Autodesk Inventor part; units mm, degrees
ref_plane "YZ Plane" through (0, 0, 0) normal (1, 0, 0) x (0, 1, 0)
ref_plane "XZ Plane" through (0, 0, 0) normal (0, 1, 0) x (-1, 0, 0)
ref_plane "XY Plane" through (0, 0, 0) normal (0, 0, 1) x (1, 0, 0)
sketch "Sketch1" plane through (0, 0, 0) normal (1, 0, 0) x (0, 1, 0)
  line L0 (0, 12.7) -> (0, -12.7)
  line L1 (0, 12.7) -> (25.4, 12.7)
  line L2 (0, -12.7) -> (25.4, -12.7)
  line L3 (25.4, 9.525) -> (3.175, 9.525)
  line L4 (3.175, 9.525) -> (3.175, -9.525)
  line L5 (3.175, -9.525) -> (25.4, -9.525)
  line L6 (25.4, 12.7) -> (25.4, 9.525)
  line L7 (25.4, -9.525) -> (25.4, -12.7)
  point P0 (0, 0)
  point P1 (0, 0)
  dimension "d0" = 25.4
  dimension "d1" = 25.4
  dimension "d2" = 25.4
  dimension "d3" = 3.175
extrude "Extrusion1" add sketch "Sketch1" along normal mid plane 64
sketch "Sketch2" plane through (-32, 3.175, 9.525) normal (0, 1, 0) x (1, 0, 0)
  circle A0 centre (4.5, 9.525) radius 3
  line L0 (0, 0) -> (0, 19.05) construction
  line L1 (0, 19.05) -> (64, 19.05) construction
  circle A1 centre (15.5, 9.525) radius 3
  circle A2 centre (26.5, 9.525) radius 3
  circle A3 centre (37.5, 9.525) radius 3
  circle A4 centre (48.5, 9.525) radius 3
  circle A5 centre (59.5, 9.525) radius 3
  point P0 (32, 9.525)
  point P1 (0, 9.525)
  point P2 (0, 9.525)
  dimension "d6" = 6
  dimension "d7" = 4.5
  dimension "d10" = 11
extrude "Extrusion2" cut sketch "Sketch2" against normal through all
sketch "Sketch3" plane through (-32, 0, 12.7) normal (0, 0, 1) x (1, 0, 0)
  line L0 (0, 3.175) -> (64, 3.175) construction
  line L1 (64, 25.4) -> (64, 3.175) construction
  line L2 (0, 25.4) -> (64, 25.4) construction
  line L3 (0, 3.175) -> (0, 25.4) construction
  circle A0 centre (4.5, 15.625) radius 3
  circle A1 centre (15.5, 15.625) radius 3
  circle A2 centre (26.5, 15.625) radius 3
  circle A3 centre (37.5, 15.625) radius 3
  circle A4 centre (48.5, 15.625) radius 3
  circle A5 centre (59.5, 15.625) radius 3
  point P0 (32, 0)
  dimension "d17" = 6
  dimension "d18" = 12.45
  dimension "d19" = 4.5
  dimension "d22" = 11
extrude "Extrusion3" cut sketch "Sketch3" against normal through all
properties part number "ArmSupport_C-Channel"
CAD build for the part. Positions are in the model's coordinates, mm. A direction names the side the tool comes from. Round coordinates to 2 decimals unless told otherwise and drop trailing zeros. Order: outer loops, then holes, each group sorted by start corner. A loop starts at its lowest first (then second) coordinate and runs counter-clockwise, first axis right, second up. Notation, with made-up numbers: (80, 14) -> (120, 14) arc R8 ccw to (120, 28) -> close; hole circle Ø9 at (87.25, 62.5). An arc over 180 degrees is marked (long way). Write item = value, one per line.
(1) Cut at A-A (z = 0). Write the cut outline in (x, y) (3 decimals).
Answers follow:
outline = (-32, 0) -> (-30.5, 0) -> (-30.5, 3.175) -> (-32, 3.175) -> close; (-24.5, 0) -> (-19.5, 0) -> (-19.5, 3.175) -> (-24.5, 3.175) -> close; (-13.5, 0) -> (-8.5, 0) -> (-8.5, 3.175) -> (-13.5, 3.175) -> close; (-2.5, 0) -> (2.5, 0) -> (2.5, 3.175) -> (-2.5, 3.175) -> close; (8.5, 0) -> (13.5, 0) -> (13.5, 3.175) -> (8.5, 3.175) -> close; (19.5, 0) -> (24.5, 0) -> (24.5, 3.175) -> (19.5, 3.175) -> close; (30.5, 0) -> (32, 0) -> (32, 3.175) -> (30.5, 3.175) -> close
(2) Drill centre lines: L1, parallel to Z at x = -25, y = 12.5 (3 decimals); L2, parallel to Y at x = -27.5, z = -12 (3 decimals); L3, parallel to Y at x = -26, z = -3.5 (3 decimals). Where is each one in solid material? Low to high.
Answers follow:
L1 = -12.7 to -9.525, 9.525 to 12.7
L2 = 0 to 12.625, 18.625 to 25.4
L3 = 0 to 3.175
(3) Cut at D-D (x = 21.5). Write the cut outline in (y, z) (3 decimals).
Answers follow:
outline = (0, -12.7) -> (25.4, -12.7) -> (25.4, -9.525) -> (3.175, -9.525) -> (3.175, 9.525) -> (25.4, 9.525) -> (25.4, 12.7) -> (0, 12.7) -> close
(4) Pull direction X, two halves, no side cores. Call faces 1 (the flat face through (0, 13, -12.7)), 2 (the flat face through (-32, 2, 0)), 3 (the flat face through (32, 2, 0)), 4 (the cylindrical face through (-19.5, 1.6, -0.1)): +X half, -X half, draft (parallel to the pull), parting line (faces both ways), or undercut.
Answers follow:
face_1 = draft
face_2 = -X half
face_3 = +X half
face_4 = undercut
(5) Cut at B-B (x = -5.5). Write the cut outline in (y, z) (3 decimals), plus the area to 3 significant figures.
Answers follow:
outline = (0, -12.7) -> (12.625, -12.7) -> (12.625, -9.525) -> (3.175, -9.525) -> (3.175, -3) -> (0, -3) -> close; (0, 3) -> (3.175, 3) -> (3.175, 9.525) -> (12.625, 9.525) -> (12.625, 12.7) -> (0, 12.7) -> close; (18.625, -12.7) -> (25.4, -12.7) -> (25.4, -9.525) -> (18.625, -9.525) -> close; (18.625, 9.525) -> (25.4, 9.525) -> (25.4, 12.7) -> (18.625, 12.7) -> close
area = 165 mm²
(6) Flat gauge pins, fed straight in: P1, Ø3.5, axis at x = -16.5, y = 15.625, coming from the +Z side; P2, Ø15, axis at x = -7.5, z = 1.5, coming from the +Y side (3 decimals). Where does each tip first touch, or does it go through?
Answers follow:
P1 = through
P2 = 3.175
(7) Cut at C-C (y = 12). Write the cut outline in (x, z) (3 decimals), plus the area to 3 significant figures.
Answers follow:
outline = (-32, -12.7) -> (32, -12.7) -> (32, -9.525) -> (-32, -9.525) -> close; (-32, 9.525) -> (32, 9.525) -> (32, 12.7) -> (-32, 12.7) -> close
area = 406 mm²
(8) 3-axis set-ups, long thin cutter, end or side, ignore diameter. For faces 5 (the cylindrical face through (4.85, 12.696, 11.135)), 6 (the flat face through (0, 14, 9.525)): which of +Z, -Z, +X, -X, +Y, -Y reach the whole face in a straight line?
Answers follow:
face_5 = +Z, -Z
face_6 = +X, -X, +Y
